from build123d import *

# Parameters (mm, degrees)
SKETCH_1_R          = 1.65
SKETCH_1_R_2        = 15
EXTRUDE_2_DEPTH     = 10
SKETCH_2_R          = 1.6
CUT_EXTRUDE_1_DEPTH = 11


with BuildPart() as part:
    # 草圖1 → 填料-伸長2 (new body)
    with BuildSketch(Plane(origin=(0, 0, 0), x_dir=(1, 0, 0), z_dir=(0, 1, 0))):
        with BuildLine():
            ThreePointArc((-17.228597844, 10.157530032), (0, -20), (17.228597844, 10.157530032))
            Line((17.228597844, 10.157530032), (102.467328593, 95.396260781))
            ThreePointArc((102.467328593, 95.396260781), (0, 140), (-102.467328593, 95.396260781))
            Line((-102.467328593, 95.396260781), (-17.228597844, 10.157530032))
        make_face()
        with Locations((-12, -13.416407865)):
            Circle(SKETCH_1_R, mode=Mode.SUBTRACT)
        Circle(SKETCH_1_R_2, mode=Mode.SUBTRACT)
        with Locations((0, 18)):
            Circle(SKETCH_1_R, mode=Mode.SUBTRACT)
        with Locations((12, -13.416407865)):
            Circle(SKETCH_1_R, mode=Mode.SUBTRACT)
        with BuildLine():
            ThreePointArc((-88.320331448, 95.39139926), (-49.748846207, 120.104339226), (-5, 129.903810568))
            Line((-5, 129.903810568), (-5, 19.364916731))
            ThreePointArc((-5, 19.364916731), (-7.653668647, 18.47759065), (-10.157530032, 17.228597844))
            Line((-10.157530032, 17.228597844), (-88.320331448, 95.39139926))
        make_face(mode=Mode.SUBTRACT)
        with BuildLine():
            Line((5, 19.364916731), (5, 129.903810568))
            ThreePointArc((5, 129.903810568), (49.748846207, 120.104339226), (88.320331448, 95.39139926))
            Line((88.320331448, 95.39139926), (10.157530032, 17.228597844))
            ThreePointArc((10.157530032, 17.228597844), (7.653668647, 18.47759065), (5, 19.364916731))
        make_face(mode=Mode.SUBTRACT)
    extrude(amount=EXTRUDE_2_DEPTH)

    # 草圖2 → 除料-伸長1 (cut, through all)
    with BuildSketch(Plane(origin=(0, 10, 0), x_dir=(1, 0, 0), z_dir=(0, 1, 0))):
        with Locations((-95.45941546, 95.45941546)):
            Circle(SKETCH_2_R)
        with Locations((0, 135)):
            Circle(SKETCH_2_R)
        with Locations((95.45941546, 95.45941546)):
            Circle(SKETCH_2_R)
    extrude(amount=-CUT_EXTRUDE_1_DEPTH, mode=Mode.SUBTRACT)


solid = part.part
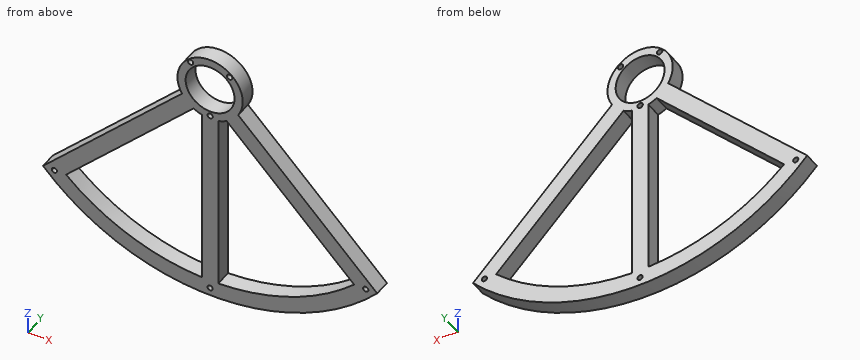
For this review, take the finished solid that the model builds, in its own axes (mm). Round coordinates to 2 decimals unless told otherwise and drop trailing zeros. Loops run counter-clockwise (first coordinate to the right, second up) from the corner with the lowest first, then second, coordinate; pieces in that order, holes last. Notation, with made-up numbers: (-33.5, 12.5) - (15.5, 12.5) arc R21 cw to (15.5, 41.5) - close; hole circle Ø8 at (-2, -35). An arc over 180 degrees is marked (long way). Answer as CSV lines item,"result".
(1) Consider section D-D on x = -85. Give the boundary of the cut face in (y, z).
Checked values:
outline,"(0, -111.24) - (10, -111.24) - (10, -98.36) - (0, -98.36) - close; (0, -92.07) - (10, -92.07) - (10, -77.93) - (0, -77.93) - close"
(2) Consider section C-C on z = -70.5. Give the boundary of the cut face in (x, y).
Checked values:
outline,"(-77.57, 0) - (-63.43, 0) - (-63.43, 10) - (-77.57, 10) - close; (-5, 0) - (5, 0) - (5, 10) - (-5, 10) - close; (63.43, 0) - (77.57, 0) - (77.57, 10) - (63.43, 10) - close"
(3) Consider section A-A on x = 31. Give the boundary of the cut face in (y, z), then the cut area to 3 significant figures.
Checked values:
outline,"(0, -136.52) - (10, -136.52) - (10, -126.25) - (0, -126.25) - close; (0, -38.07) - (10, -38.07) - (10, -23.93) - (0, -23.93) - close"
area,"244 mm2"
(4) Insertion check: P1, Ø10, axis at x = -48.5, z = -119, coming from the +Y side; P2, Ø12, axis at x = 4.5, z = 2.5, coming from the +Y side; P3, Ø3, axis at y = 3, z = -55.5, coming from the -X side; P4, Ø2, axis at x = 63.5, y = 5.5, coming from the +Z side. Each pin has a flat end and moves straight along its axis. Give the tip position at first contact, or say it passes through.
Checked values:
P1,"stops at y = 10"
P2,"passes through"
P3,"stops at x = -64.07"
P4,"stops at z = -55.43"
(5) Consider section B-B on y = 8. Give the number of separate pieces and of enclosed holes in the cut face, then the cut area to 3 significant figures.
Checked values:
separate pieces,"1"
enclosed holes,"9"
area,"6,030 mm2"
(6) Wall thickness on line 1 (Z direction, x = 0, y = 6.75); line 2 (Z direction, x = 18, y = 2); line 3 (X direction, y = 3.25, z = -35): over which ranges is each line inside the solid? List them lowest first.
Checked values:
line 1,"z = -140 to -136.6, -133.4 to -19.65, -16.35 to -15, 15 to 20"
line 2,"z = -138.84 to -128.75, -25.07 to -10.93, -8.72 to 8.72"
line 3,"x = -42.07 to -27.93, -5 to 5, 27.93 to 42.07"
